```python
from build123d import *

# Parameters (mm, degrees)
BOSS_EXTRUDE1_DEPTH        = 31.75
FILLET1_R                  = 6.35
SHELL1_T                   = -3.175
F_9_0_196_DIAMETER_HOLE1_D = 4.9784
F_9_0_196_DIAMETER_HOLE2_D = 4.9784
CHAMFER1_SIZE              = 1.905
FILLET2_R                  = 1.27


with BuildPart() as part:
    # Sketch1 → Boss-Extrude1 (new body)
    with BuildSketch(Plane(origin=(0, 0, 0), x_dir=(1, 0, 0), z_dir=(0, 1, 0))):
        Polygon((0, 0), (0, -38.1), (-12.7, -38.1), (-12.7, -12.7), (-50.8, -12.7), (-50.8, 0), align=None)
    extrude(amount=BOSS_EXTRUDE1_DEPTH)

    # Fillet1
    fillet1_edges = [part.edges().sort_by_distance(p)[0] for p in [
        (0, 15.875, 0),
        (-12.7, 15.875, 12.7),
    ]]
    fillet(fillet1_edges, radius=FILLET1_R)

    # Shell1
    shell1_openings = [part.faces().sort_by_distance(p)[0] for p in [
        (-6.35, 15.875, 38.1),
        (-50.8, 15.875, 6.35),
        (-18.721217985, 0, 15.546217985),
    ]]
    offset(amount=SHELL1_T, openings=shell1_openings, kind=Kind.INTERSECTION)

    # #9 (0.196) Diameter Hole1 (through all)
    with Locations(Plane.ZY.offset(12.7)):
        with Locations((25.4, 15.875)):
            Hole(F_9_0_196_DIAMETER_HOLE1_D / 2)

    # #9 (0.196) Diameter Hole2 (through all)
    with Locations(Plane.XY.offset(12.7)):
        with Locations((-38.1, 15.875)):
            Hole(F_9_0_196_DIAMETER_HOLE2_D / 2)

    # Chamfer1
    chamfer1_edges = [part.edges().sort_by_distance(p)[0] for p in [
        (-28.575, 0, 3.175),
        (-34.925, 0, 9.525),
        (-9.525, 0, 28.575),
        (-3.175, 0, 22.225),
        (-4.10493597, 0, 4.10493597),
        (-12.314807909, 0, 12.314807909),
    ]]
    chamfer(chamfer1_edges, length=CHAMFER1_SIZE)

    # Fillet2
    fillet2_edges = [part.edges().sort_by_distance(p)[0] for p in [
        (-34.925, 31.75, 12.7),
        (-28.575, 31.75, 0),
        (-12.7, 31.75, 28.575),
        (-1.859871939, 31.75, 1.859871939),
        (0, 31.75, 22.225),
        (-14.559871939, 31.75, 14.559871939),
        (-3.175, 28.575, 22.225),
        (-4.10493597, 28.575, 4.10493597),
        (-28.575, 28.575, 3.175),
        (-34.925, 28.575, 9.525),
        (-12.314807909, 28.575, 12.314807909),
        (-9.525, 28.575, 28.575),
    ]]
    fillet(fillet2_edges, radius=FILLET2_R)


solid = part.part
```
Work out the finished part from the listing and answer in its coordinate system (mm). A direction names the side the tool comes from. Give positions to 0.01 mm unless a question says otherwise; leave off trailing zeros. Write each loop counter-clockwise with the first axis right and the second up, starting at its lowest first coordinate (ties: lowest second). Pieces come first, ordered by that corner, then holes.
(1) The part is cut by section A-A on z = 25.4. Write down the section's boundary in (x, y) (3 decimals).
Final values:
outline: (-12.7, 0) - (-11.43, 0) - (-9.525, 1.905) - (-9.525, 13.386) - (-12.7, 13.386) - close; (-12.7, 18.364) - (-9.525, 18.364) - (-9.525, 27.305) arc R1.27 cw to (-8.255, 28.575) - (-4.445, 28.575) arc R1.27 cw to (-3.175, 27.305) - (-3.175, 18.364) - (0, 18.364) - (0, 30.48) arc R1.27 ccw to (-1.27, 31.75) - (-11.43, 31.75) arc R1.27 ccw to (-12.7, 30.48) - close; (-3.175, 1.905) - (-1.27, 0) - (0, 0) - (0, 13.386) - (-3.175, 13.386) - close
(2) The part is cut by section C-C on y = 23.5. Write down the section's boundary in (x, z) (3 decimals), plus the area to 3 significant figures.
Final values:
outline: (-50.8, 0) - (-6.35, 0) arc R6.35 ccw to (0, 6.35) - (0, 38.1) - (-3.175, 38.1) - (-3.175, 6.35) arc R3.175 cw to (-6.35, 3.175) - (-50.8, 3.175) - close; (-50.8, 9.525) - (-19.05, 9.525) arc R9.525 ccw to (-9.525, 19.05) - (-9.525, 38.1) - (-12.7, 38.1) - (-12.7, 19.05) arc R6.35 cw to (-19.05, 12.7) - (-50.8, 12.7) - close
area: 467 mm2
(3) Which of the six approach directions +Z, -Z, +X, -X, +Y, -Y give full straight-line access (tool end or side, diameter ignored) to faces 4 (the cylindrical face through (-35.147, 31.388, 12.318)), 5 (the flat face through (-35, 15, 12.7)), 6 (the flat face through (-3.175, 14, 22)), 7 (the flat face through (-34.7, 0.97, 10.46)), 8 (the cylindrical face through (-12.24, 14.78, 12.39))?
Final values:
face 4: +Z, -X, +Y
face 5: +Z, -X, +Y, -Y
face 6: +Z, -Y
face 7: -X, -Y
face 8: -Y
(4) Straight lines are drawn through the part: line 1 (Z direction, x = -25.5, y = 20) (3 decimals); line 2 (X direction, y = 19.5, z = 21.5) (3 decimals); line 3 (Y direction, x = -38.1, z = 1.25). For each, find the intervals that lie inside material, in ascending order.
Final values:
line 1: z = 0 to 3.175, 9.525 to 12.7
line 2: x = -12.7 to -9.525, -3.175 to 0
line 3: y = 0 to 13.39, 18.36 to 31.75
(5) Flat-ended cylindrical pins translate along their axes: pin 1 Ø5 at (x, z) = (-14, 25.5) entering from +Y; pin 2 Ø10 at (x, z) = (-20, 23.5) entering from -Y; pin 3 Ø5.5 at (y, z) = (15.875, 25.4) entering from -X; pin 4 Ø7.5 at (x, y) = (-38.5, 16) entering from +Z. Find the tip coordinate at first contact, or state that the pin passes through.
Final values:
pin 1: stops at y = 31.75
pin 2: passes through
pin 3: stops at x = -12.7
pin 4: stops at z = 12.7
(6) The part is cut by section B-B on x = -38.1. Write down the section's boundary in (y, z) (3 decimals).
Final values:
outline: (0, 0) - (13.386, 0) - (13.386, 3.175) - (1.905, 3.175) - (0, 1.27) - close; (0, 11.43) - (1.905, 9.525) - (13.386, 9.525) - (13.386, 12.7) - (0, 12.7) - close; (18.364, 0) - (30.48, 0) arc R1.27 ccw to (31.75, 1.27) - (31.75, 11.43) arc R1.27 ccw to (30.48, 12.7) - (18.364, 12.7) - (18.364, 9.525) - (27.305, 9.525) arc R1.27 cw to (28.575, 8.255) - (28.575, 4.445) arc R1.27 cw to (27.305, 3.175) - (18.364, 3.175) - close
(7) The mould has two halves that part along X. Classify faces 1 (the cylindrical face through (-14.51, 15.45, 14.61)), 2 (the flat face through (-20, 31.75, 11)), 3 (the cylindrical face through (-3.557, 28.213, 22.003)): pulls with the +X half, pulls with the -X half, needs draft (parallel to the pull), parting line crosses it, or undercut.
Final values:
face 1: pulls with the -X half
face 2: needs draft
face 3: undercut
(8) The part is cut by section D-D on x = -43.5. Write down the section's boundary in (y, z) (3 decimals), plus the area to 3 significant figures.
Final values:
outline: (0, 0) - (30.48, 0) arc R1.27 ccw to (31.75, 1.27) - (31.75, 11.43) arc R1.27 ccw to (30.48, 12.7) - (0, 12.7) - (0, 11.43) - (1.905, 9.525) - (27.305, 9.525) arc R1.27 cw to (28.575, 8.255) - (28.575, 4.445) arc R1.27 cw to (27.305, 3.175) - (1.905, 3.175) - (0, 1.27) - close
area: 218 mm2
